from build123d import *

# Parameters (mm, degrees)
SKETCH8_R           = 2.286
BOSS_EXTRUDE1_DEPTH = 12.7
SKETCH9_R           = 1.905
CUT_EXTRUDE4_DEPTH  = 15.875
CUT_EXTRUDE5_DEPTH  = 65.018582459
SKETCH11_R          = 4.064
CUT_EXTRUDE6_DEPTH  = 6.35
FILLET1_R           = 3.81
FILLET2_R           = 0.79375


with BuildPart() as part:
    # Sketch8 → Boss-Extrude1 (new body)
    with BuildSketch(Plane.XY):
        Polygon((0, 0), (-25.4, 0), (-50.8, 24.13), (-50.8, 36.83), (-38.1, 36.83), (0, 14.832954744), align=None)
        with Locations((-12.7, 11.826875)):
            Circle(SKETCH8_R, mode=Mode.SUBTRACT)
        with Locations((-46.0375, 32.0675)):
            Circle(SKETCH8_R, mode=Mode.SUBTRACT)
    extrude(amount=BOSS_EXTRUDE1_DEPTH)

    # Sketch9 → Cut-Extrude4 (cut)
    with BuildSketch(Plane.XZ):
        with Locations((-6.35, 6.35)):
            Circle(SKETCH9_R)
        with Locations((-19.05, 6.35)):
            Circle(SKETCH9_R)
    extrude(amount=-CUT_EXTRUDE4_DEPTH, mode=Mode.SUBTRACT)

    # Sketch10 → Cut-Extrude5 (cut, through all)
    with BuildSketch(Plane.ZY.offset(50.8)):
        Polygon((6.35, 36.83), (6.35, 24.13), (12.7, 6.35), (12.7, 36.83), align=None)
    extrude(amount=-CUT_EXTRUDE5_DEPTH, mode=Mode.SUBTRACT)

    # Sketch11 → Cut-Extrude6 (cut)
    with BuildSketch(Plane.XY.offset(12.7)):
        with Locations(Location((-12.7, 11.826875, 0), (0, 0, 270))):
            Circle(SKETCH11_R)
    extrude(amount=-CUT_EXTRUDE6_DEPTH, mode=Mode.SUBTRACT)

    # Fillet1
    fillet1_edges = [part.edges().sort_by_distance(p)[0] for p in [
        (-50.8, 24.13, 3.175),
        (-50.8, 36.83, 3.175),
        (-38.1, 36.83, 3.175),
        (0, 14.832954744, 4.835186653),
    ]]
    fillet(fillet1_edges, radius=FILLET1_R)

    # Fillet2
    fillet2_edges = [part.edges().sort_by_distance(p)[0] for p in [
        (0, 0, 6.35),
        (-25.4, 0, 6.35),
        (-12.7, 0, 12.7),
        (-28.742105263, 3.175, 12.7),
        (-9.003977372, 20.031403503, 7.813784463),
        (-16.042105263, 6.35, 12.7),
        (-40.849172988, 14.676714339, 9.72617345),
        (-33.266990546, 24.13, 6.35),
        (0, 3.175, 12.7),
        (-12.7, 0, 0),
        (-12.699987477, 15.890875, 9.292544643),
        (-37.507067725, 11.501714339, 0),
        (-50.8, 29.39283826, 0),
        (-43.055443212, 36.83, 0),
        (-19.560443212, 26.126181898, 0),
        (-0.510443212, 14.538250218, 0),
        (-38.134785861, 36.700177398, 0),
        (-49.684076836, 35.714076836, 0),
        (-50.491003861, 24.262655572, 0),
        (-50.8, 29.39283826, 6.35),
        (-43.055443212, 36.83, 6.35),
        (-26.659420584, 30.224778394, 6.35),
        (-38.134785861, 36.700177398, 6.35),
        (-49.684076836, 35.714076836, 6.35),
        (-50.706612058, 24.927288299, 6.35),
        (0, 9.491625109, 11.577991032),
        (0, 6.316625109, 0),
        (-0.498461944, 14.517345679, 9.783090829),
        (-50.076536566, 23.531981816, 6.563577923),
    ]]
    fillet(fillet2_edges, radius=FILLET2_R)


solid = part.part
Geometry: final body of the model. Coordinates: model frame, mm. A direction names the side the tool comes from. Round coordinates to 2 decimals unless told otherwise and drop trailing zeros. Loops run counter-clockwise (first coordinate to the right, second up) from the corner with the lowest first, then second, coordinate; pieces in that order, holes last. Notation, with made-up numbers: (61.5, 31) - (72.5, 31) arc R21 ccw to (72.5, 62) - close; hole circle Ø1 at (-20, 11). An arc over 180 degrees is marked (long way). Write each question's results on one line, items separated by ' | '. Start each with the question number.
1) Cut plane A-A on z = 1.5. Return loops of the section in (x, y) (1 decimal).
2) First-contact query: P1, Ø7.5, axis at x = -12.7, y = 11.83, coming from the +Z side; P2, Ø1.9, axis at x = -19, z = 6, coming from the -Y side (3 decimals); P3, Ø5, axis at x = -33.5, y = 9.5, coming from the +Z side. Flat tips, straight axial feed; report the tip coordinate or a pass-through.
3) Line query: probe 1 along Z at (x, y) = (-6.35, 4.5) (3 decimals); probe 2 along X at (y, z) = (13, 7); probe 3 along X at (y, z) = (8.5, 7.5). Output: solid intervals per line, ascending. Write a range as [from, to].
4) Access query for faces 1 (the face through (-37.63, 11.94, 0.23)), 2 (the face through (-17.3, 7.8, 5.6)), 3 (the face through (-38, 29, 6.35)). Directions: +Z, -Z, +X, -X, +Y, -Y. A direction counts if a zero-diameter tool reaches every point of the face in a straight line with its end or side. Return the directions, or none.
5) Mould query, pull axis X, two halves, no side actions, for faces 4 (the face through (-19.43, 25.78, 0.23)), 5 (the face through (-43, 36.83, 3)), 6 (the face through (-14.45, 10.08, 6.35)). Classes: released by +X, released by -X, zero draft, split by the parting line, or undercut.
Verdict:
1) outline: (-50.8, 25.8) arc R3.8 ccw to (-49.6, 23) - (-25.6, 0.2) arc R0.8 ccw to (-25.1, 0) - (-0.8, 0) arc R0.8 ccw to (0, 0.8) - (0, 12.6) arc R3.8 ccw to (-1.9, 15.9) - (-37.2, 36.3) arc R3.8 ccw to (-39.1, 36.8) - (-47, 36.8) arc R3.8 ccw to (-50.8, 33) - close; hole circle Ø4.6 at (-46, 32.1); hole circle Ø4.6 at (-12.7, 11.8)
2) P1: stops at z = 6.35 | P2: stops at y = 15.875 | P3: stops at z = 12.29
3) probe 1: z = [0, 4.445], [8.255, 12.7] | probe 2: x = [-39.08, -20.84], [-17.26, -16.59], [-8.81, -8.14], [-4.56, -0.02] | probe 3: x = [-34.35, -20.57], [-17.53, -15.03], [-10.37, -7.87], [-4.83, 0]
4) face 1: -Z, -X, -Y | face 2: -Y | face 3: +Z, +X, -X, +Y
5) face 4: released by +X | face 5: zero draft | face 6: undercut
